```python
from build123d import *

# Parameters (mm, degrees)
SKETCH_1_W                  = 10
SKETCH_1_H                  = 10
SKETCH_6_R                  = 14
SKETCH_6_R_2                = 12
EXTRUDE_1_DEPTH             = 3
SKETCH_7_R                  = 19.5
EXTRUDE_2_DEPTH             = 10
HOLE_WIZARD_M43_D           = 3.3
HOLE_WIZARD_M43_DEPTH       = 12
HOLE_WIZARD_M43_CSINK_D     = 5
HOLE_WIZARD_M43_CSINK_ANGLE = 90
HOLE_WIZARD_M43_TIP         = 0.991420021
EXTRUDE_START               = -10
EXTRUDE_3_DEPTH             = 10
HOLE_WIZARD_M61_D           = 6.5
CHAMFER_1_SIZE              = 1


with BuildPart() as part:
    # Эскиз1 → Повернуть1 (revolve)
    with BuildSketch(Plane.XY, mode=Mode.PRIVATE) as revolve_1_sk:
        with Locations((5, 19)):
            Rectangle(SKETCH_1_W, SKETCH_1_H)
    revolve(revolve_1_sk.sketch.rotate(Axis((-29.36512031, 0, 0), (1, 0, 0)), 90), axis=Axis((-29.36512031, 0, 0), (1, 0, 0)))

    # Эскиз6 → Бобышка-Вытянуть1 (add)
    with BuildSketch(Plane.ZY):
        Circle(SKETCH_6_R)
        Circle(SKETCH_6_R_2, mode=Mode.SUBTRACT)
    extrude(amount=-EXTRUDE_1_DEPTH)

    # Эскиз7 → Бобышка-Вытянуть2 (add)
    with BuildSketch(Plane.ZY):
        with BuildLine():
            Line((-30.415116076, -30), (30.415116076, -30))
            ThreePointArc((30.415116076, -30), (34.632073305, -27.686498042), (34.946655011, -22.886908691))
            Line((34.946655011, -22.886908691), (19.938771315, 9.297601758))
            ThreePointArc((19.938771315, 9.297601758), (0, 22), (-19.938771315, 9.297601758))
            Line((-19.938771315, 9.297601758), (-34.946655011, -22.886908691))
            ThreePointArc((-34.946655011, -22.886908691), (-34.632073305, -27.686498042), (-30.415116076, -30))
        make_face()
        Circle(SKETCH_7_R, mode=Mode.SUBTRACT)
    extrude(amount=-EXTRUDE_2_DEPTH)

    # Отверстие обработанное метчиком M43
    with Locations(Plane(origin=(0, -30, 0), x_dir=(-1, 0, 0), z_dir=(0, -1, 0))):
        with Locations((-5, 0), (-5, 25), (-5, -25)):
            CounterSinkHole(HOLE_WIZARD_M43_D / 2, HOLE_WIZARD_M43_CSINK_D / 2, depth=HOLE_WIZARD_M43_DEPTH, counter_sink_angle=HOLE_WIZARD_M43_CSINK_ANGLE)
            with Locations((0, 0, -(HOLE_WIZARD_M43_DEPTH + HOLE_WIZARD_M43_TIP / 2))):  # 118° drill point
                Cone(0, HOLE_WIZARD_M43_D / 2, HOLE_WIZARD_M43_TIP, mode=Mode.SUBTRACT)

    # Эскиз10 → Бобышка-Вытянуть3 (add)
    with BuildSketch(Plane.ZY.offset(EXTRUDE_START)):
        with BuildLine():
            Line((-12.507364702, 20.483306086), (-5.543277195, 37.296100594))
            ThreePointArc((-5.543277195, 37.296100594), (0, 41), (5.543277195, 37.296100594))
            Line((5.543277195, 37.296100594), (12.507364702, 20.483306086))
            ThreePointArc((12.507364702, 20.483306086), (0, 24), (-12.507364702, 20.483306086))
        make_face()
    extrude(amount=EXTRUDE_3_DEPTH)

    # Сверло под метчик  спиральное M61 (through all)
    with Locations(Plane.ZY):
        with Locations((0, 35)):
            Hole(HOLE_WIZARD_M61_D / 2)

    # Фаска1
    chamfer_1_edges = [part.edges().sort_by_distance(p)[0] for p in [
        (10, 0, -14),
    ]]
    chamfer(chamfer_1_edges, length=CHAMFER_1_SIZE)


solid = part.part
```
Could you check a few things on this model? Use its own coordinates, in mm. A direction names the side the tool comes from. Round coordinates to 2 decimals unless told otherwise and drop trailing zeros. Write each loop counter-clockwise with the first axis right and the second up, starting at its lowest first coordinate (ties: lowest second). Pieces come first, ordered by that corner, then holes.
(1) Suppose I cut it at A-A on y = 18. Write out the boundary of the cut face in (x, z), and give its area (3 significant figures).
Findings below:
outline: (0, -15.87) - (10, -15.87) - (10, 15.87) - (0, 15.87) - close
area: 317 mm2
(2) Thinking about a two-plate mould opening in X: for faces 4 (the face through (5.04, -17.18, -25.28)), 5 (the face through (5.07, 31.827, 0.705)), 6 (the face through (0, -10, 7)), which applies, +X half, -X half, draft (parallel to the pull), parting line (faces both ways), or undercut?
Findings below:
face 4: undercut
face 5: draft
face 6: -X half
(3) If I drill on probe 1 along Y at (x, z) = (1.8, 0); probe 2 along Y at (x, z) = (5.75, 0); probe 3 along X at (y, z) = (-23.75, 25), over which ranges is the centre line in solid material (lowest first)?
Findings below:
probe 1: y = -30 to -12, 12 to 31.75, 38.25 to 41
probe 2: y = -17.46 to -14, 14 to 31.75, 38.25 to 41
probe 3: x = 0 to 3.35, 6.65 to 10
(4) Which directions (+Z, -Z, +X, -X, +Y, -Y) give clear straight access to the entire face, cutting with the end or side of a thin tool? Please do faces 1 (the face through (6, 12.4, 6.5)), 2 (the face through (4.785, -23.497, 23.364)), 3 (the face through (4.93, -27.627, -34.669)).
Findings below:
face 1: +X
face 2: -Y
face 3: -Z, +X, -X
(5) For pin 1 (1 mm diameter, centred on y = 8.5, z = 9.5, fed in from +X); pin 2 (1.5 mm diameter, centred on x = 4.5, y = 27.5, fed in from -Z); pin 3 (1 mm diameter, centred on x = 2, y = -21.5, fed in from -Z); pin 4 (5 mm diameter, centred on y = 35, z = 0, fed in from +X), each with a flat end and sliding along its axis, tell me the tip position at first contact or that it passes through.
Findings below:
pin 1: stops at x = 3
pin 2: stops at z = -9.91
pin 3: stops at z = -34.53
pin 4: passes through
